Geometry: see drawing. Coordinates: mm, zero at the bounding-box minimum. A direction names the side the tool comes from. Give positions to 0.01 mm unless a question says otherwise; leave off trailing zeros. Write each loop counter-clockwise with the first axis right and the second up, starting at its lowest first coordinate (ties: lowest second). Pieces come first, ordered by that corner, then holes. Notation, with made-up numbers: M 12.25,43.25 L 55.25,43.25 A29 ccw 55.25,63.25 Z; hole C 44.25,24.5 d11. An arc over 180 degrees is marked long. Use a Markdown table: item, result. Add a question column.
1) Section A-A on y = 67. Return the cut outline in (x, z), then the cut area to 3 significant figures.
2) Section B-B on x = 28. Return the cut outline in (y, z), then the cut area to 3 significant figures.
3) Section C-C on z = 9. Return the cut outline in (x, y), then the cut area to 3 significant figures.
4) Line query: line 1 (Z direction, x = 51.35, y = 67); line 2 (Y direction, x = 28, z = 1); line 3 (X direction, y = 14, z = 31). Output: solid intervals per line, ascending.
5) Pin query (flat end, axial travel): pin 1 (5.5 mm diameter, centred on y = 6, z = 55, fed in from -X); pin 2 (2.5 mm diameter, centred on x = 16.69, y = 37.69, fed in from +Z); pin 3 (2 mm diameter, centred on x = 29, y = 32.5, fed in from +Z). Return the tip coordinate at first contact, or that it passes through.
6) Section D-D on y = 47.5. Return the cut outline in (x, z), then the cut area to 3 significant figures.
7) Set-up query: the marked faces 1 and 2. Return all of +Z, -Z, +X, -X, +Y, -Y with unobstructed straight access to the full face (end or side cutting, diameter ignored); none if empty.
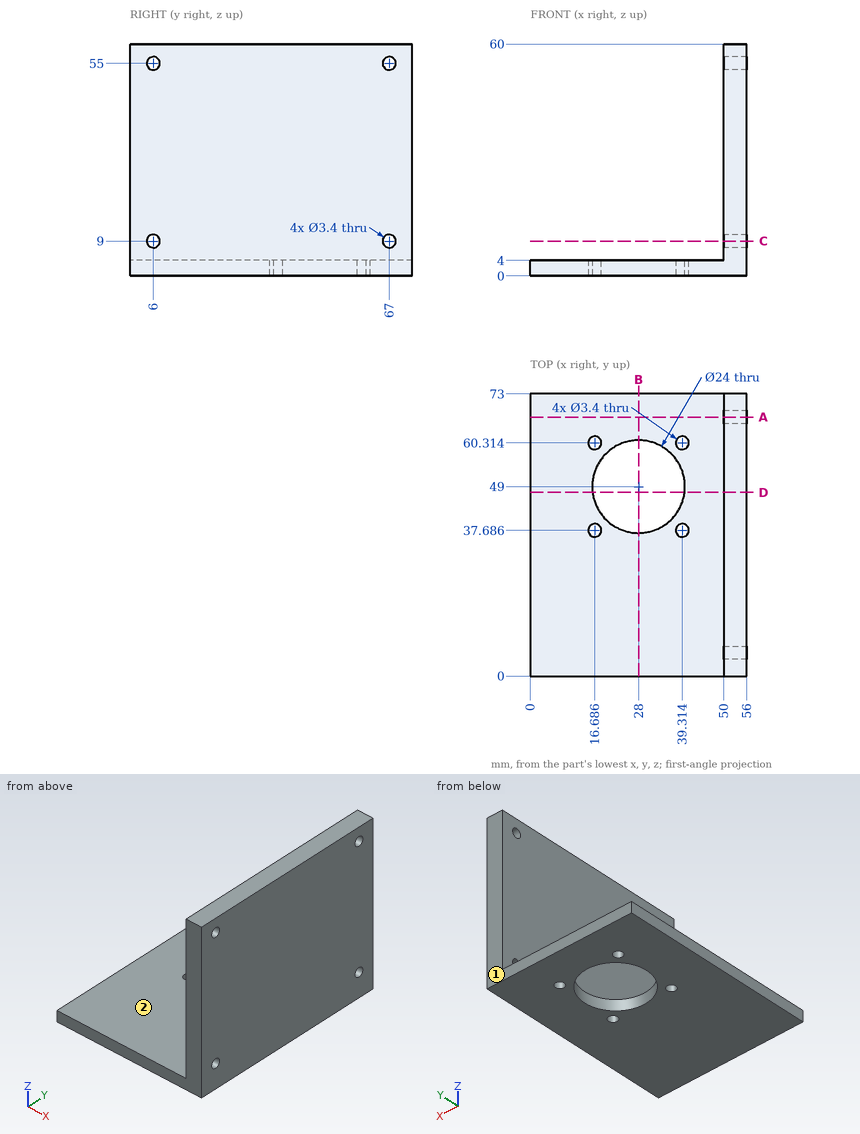
Found:
| question | item | result |
|---|---|---|
| 1 | outline | M 0,0 L 56,0 L 56,7.3 L 50,7.3 L 50,4 L 0,4 Z; M 50,10.7 L 56,10.7 L 56,53.3 L 50,53.3 Z; M 50,56.7 L 56,56.7 L 56,60 L 50,60 Z |
| 1 | area | 519 mm² |
| 2 | outline | M 0,0 L 37,0 L 37,4 L 0,4 Z; M 61,0 L 73,0 L 73,4 L 61,4 Z |
| 2 | area | 196 mm² |
| 3 | outline | M 50,0 L 56,0 L 56,4.3 L 50,4.3 Z; M 50,7.7 L 56,7.7 L 56,65.3 L 50,65.3 Z; M 50,68.7 L 56,68.7 L 56,73 L 50,73 Z |
| 3 | area | 397 mm² |
| 4 | line 1 | 0 to 7.3, 10.7 to 53.3, 56.7 to 60 |
| 4 | line 2 | 0 to 37, 61 to 73 |
| 4 | line 3 | 50 to 56 |
| 5 | pin 1 | x = 50 |
| 5 | pin 2 | through |
| 5 | pin 3 | z = 4 |
| 6 | outline | M 0,0 L 16.09,0 L 16.09,4 L 0,4 Z; M 39.91,0 L 56,0 L 56,60 L 50,60 L 50,4 L 39.91,4 Z |
| 6 | area | 465 mm² |
| 7 | face 1 | +Z, -Z, +X, -X, +Y |
| 7 | face 2 | +Z, -X, +Y, -Y |
